from build123d import *

# Parameters (mm, degrees)
SKETCH_R              = 66
PAD_DEPTH             = 7
SKETCH001_R           = 30
PAD001_DEPTH          = 15
PAD002_DEPTH          = 15
POCKET_DEPTH          = 7
POLARPATTERN_COUNT    = 4
FILLET_R              = 10
FILLET001_R           = 2
SKETCH004_R           = 6
POCKET001_DEPTH       = 37.001
SKETCH005_R           = 23
POCKET002_DEPTH       = 10
SKETCH006_R           = 4
POCKET003_DEPTH       = 4
POLARPATTERN001_COUNT = 4
SKETCH007_R           = 2.25
POCKET004_DEPTH       = 535.079942
POLARPATTERN002_COUNT = 4
CHAMFER_SIZE          = 1
SKETCH008_R           = 4
POCKET005_DEPTH       = 37.001


with BuildPart() as part:
    # Sketch → Pad (new body)
    with BuildSketch(Plane.XY):
        Circle(SKETCH_R)
    extrude(amount=PAD_DEPTH)

    # Sketch001 (on Face3 of Pad) → Pad001 (join)
    with BuildSketch(Plane.XY.offset(7)):
        Circle(SKETCH001_R)
    extrude(amount=PAD001_DEPTH)

    # Sketch002 (on Face5 of Pad001) → Pad002 (join)
    with BuildSketch(Plane.XY.offset(22)):
        with BuildLine():
            ThreePointArc((0.3, 14.997), (-15, 0), (0.3, -14.997))
            Line((0.3, -14.997), (150.24, -11.9976))
            ThreePointArc((150.24, -11.9976), (162, 0), (150.24, 11.9976))
            Line((0.3, 14.997), (150.24, 11.9976))
        make_face()
    extrude(amount=PAD002_DEPTH)

    # Sketch003 (on Face3 of Pad002) → Pocket (cut)
    with BuildSketch(Plane.XY.offset(7)):
        with BuildLine():
            ThreePointArc((-6, 49.638695), (-35.355339, 35.355339), (-49.638695, 6))
            Line((-33.76825, 6), (-49.638695, 6))
            ThreePointArc((-6, 33.636641), (-24.113209, 24.067543), (-33.76825, 6))
            Line((-6, 33.636641), (-6, 49.638695))
        make_face()
    pocket = extrude(amount=-POCKET_DEPTH, mode=Mode.SUBTRACT)

    # PolarPattern: Pocket ×4 about axis
    polarpattern_axis = Axis((0, 0, 0), (0, 0, 1))
    for i in range(1, POLARPATTERN_COUNT):
        add(pocket.rotate(polarpattern_axis, i * 360 / POLARPATTERN_COUNT), mode=Mode.SUBTRACT)

    # Fillet
    fillet_edges = [part.edges().sort_by_distance(p)[0] for p in [
        (-30, 0, 22),
    ]]
    fillet(fillet_edges, radius=FILLET_R)

    # Fillet001
    fillet001_edges = [part.edges().sort_by_distance(p)[0] for p in [
        (-33.636641, -6, 3.5),
        (-49.638695, -6, 3.5),
        (-66, 0, 7),
        (-49.638695, 6, 3.5),
        (-6, 49.638695, 3.5),
        (-6, -33.76825, 3.5),
        (-6, -49.638695, 3.5),
        (6, -49.638695, 3.5),
        (6, -33.636641, 3.5),
        (33.76825, -6, 3.5),
        (49.638695, -6, 3.5),
        (49.638695, 6, 3.5),
        (6, 49.638695, 3.5),
        (6, 33.76825, 3.5),
        (33.636641, 6, 3.5),
        (-6, 33.636641, 3.5),
        (-33.76825, 6, 3.5),
        (75.27, -13.4973, 37),
        (-15, 0, 37),
        (75.27, 13.4973, 37),
        (162, 0, 37),
        (88.257783, 13.237492, 22),
        (162, 0, 22),
        (88.257783, -13.237492, 22),
        (-30, 0, 12),
    ]]
    fillet(fillet001_edges, radius=FILLET001_R)

    # Sketch004 (on Face50 of Fillet001) → Pocket001 (cut, through all)
    with BuildSketch(Plane.XY.offset(37)):
        Circle(SKETCH004_R)
    extrude(amount=-POCKET001_DEPTH, mode=Mode.SUBTRACT)

    # Sketch005 (on Face51 of Pocket001) → Pocket002 (cut)
    with BuildSketch(Plane(origin=(0, 0, 0), x_dir=(1, 0, 0), z_dir=(0, 0, -1))):
        with Locations((0.306212, -0.34782)):
            Circle(SKETCH005_R)
    extrude(amount=-POCKET002_DEPTH, mode=Mode.SUBTRACT)

    # Sketch006 (on Face5 of Pocket002) → Pocket003 (cut)
    with BuildSketch(Plane.XY.offset(7)):
        with Locations((-42.376377, 42.476376)):
            Circle(SKETCH006_R)
    pocket003 = extrude(amount=-POCKET003_DEPTH, mode=Mode.SUBTRACT)

    # PolarPattern001: Pocket003 ×4 about axis
    polarpattern001_axis = Axis((0, 0, 0), (0, 0, 1))
    for i in range(1, POLARPATTERN001_COUNT):
        add(pocket003.rotate(polarpattern001_axis, i * 360 / POLARPATTERN001_COUNT), mode=Mode.SUBTRACT)

    # Sketch007 (on Face57 of PolarPattern001) → Pocket004 (cut, through all)
    with BuildSketch(Plane.XY.offset(3)):
        with Locations((-42.376377, 42.476376)):
            Circle(SKETCH007_R)
    pocket004 = extrude(amount=-POCKET004_DEPTH, mode=Mode.SUBTRACT)

    # PolarPattern002: Pocket004 ×4 about axis
    polarpattern002_axis = Axis((0, 0, 0), (0, 0, 1))
    for i in range(1, POLARPATTERN002_COUNT):
        add(pocket004.rotate(polarpattern002_axis, i * 360 / POLARPATTERN002_COUNT), mode=Mode.SUBTRACT)

    # Chamfer
    chamfer_edges = [part.edges().sort_by_distance(p)[0] for p in [
        (-6, 0, 37),
    ]]
    chamfer(chamfer_edges, length=CHAMFER_SIZE)

    # Sketch008 (on Face1 of Chamfer) → Pocket005 (cut, through all)
    with BuildSketch(Plane.XY.offset(37)):
        with Locations((150, 0)):
            Circle(SKETCH008_R)
    extrude(amount=-POCKET005_DEPTH, mode=Mode.SUBTRACT)


solid = part.part
Verification items for the finished model (mm, model axes). A direction names the side the tool comes from. Coordinates: 2 decimals unless noted, no trailing zeros. Write each loop counter-clockwise with the first axis right and the second up, starting at its lowest first coordinate (ties: lowest second). Pieces come first, ordered by that corner, then holes. Notation, with made-up numbers: (64, -11) -> (114, -11) arc R19 ccw to (114, 8) -> close; hole circle Ø2 at (41.5, -19). An arc over 180 degrees is marked (long way). One line per item, written item: value. Start each with the question number.
Q1. Go/stop test with flat-tipped pins: P1, Ø1.5, axis at x = 47.5, y = 22.5, coming from the +Z side; P2, Ø8, axis at y = 6, z = 24.5, coming from the -X side; P3, Ø7, axis at x = 42.48, y = 42.38, coming from the +Z side; P4, Ø8, axis at x = -40.5, z = 14.5, coming from the +Y side. Record where each tip stops, or that it passes through.
Q2. Cross-section at A-A on z = 27.5. Enter the section's corners in (x, y), and give its area (3 significant figures).
Q3. Thickness scan on L1, parallel to X at y = -17, z = 4; L2, parallel to Y at x = 150, z = 31.25; L3, parallel to X at y = 7, z = 5. Record the ranges inside material, lowest first. Write a range as from..to.
Q4. Access from +Z, -Z, +X, -X, +Y, -Y to the whole of each face (thin tool, end or side, straight path). Record for faces 1 (the flat face through (-6, 41, 4)), 2 (the flat face through (-40.65, 40.75, 3)), 3 (the cylindrical face through (74.208, 12.917, 36.43)), 4 (the cylindrical face through (-4.68, 22.8, 4.93)).
Q5. Mould release check, pull along Z, two halves, no side actions. Record for faces 5 (the flat face through (72, 0, 37)), 6 (the flat face through (93, 0, 22)), 7 (the cylindrical face through (-35.66, -35.05, 3.55)): pulls with the +Z half, pulls with the -Z half, needs draft (parallel to the pull), parting line crosses it, or undercut.
Checked values:
1. P1: stops at z = 7
1. P2: stops at x = -24.61
1. P3: stops at z = 3
1. P4: passes through
2. outline: (0.3, -15) -> (150.24, -12) arc R12 ccw to (150.24, 12) -> (0.3, 15) arc R15 ccw (long way) to start; hole circle Ø12 at (0, 0); hole circle Ø8 at (150, 0)
2. area: 4,470 mm²
3. L1: x = -63.77..-47.02, -29.53..-14.8, 15.41..29.59, 47.02..63.77
3. L2: y = -12..-4, 4..12
3. L3: x = -65.63..-49.06, -33.64..-21.71, 22.32..33.52, 49.06..65.63
4. face 1: +Z, -Z
4. face 2: +Z
4. face 3: +Z, +X, +Y
4. face 4: -Z
5. face 5: pulls with the +Z half
5. face 6: undercut
5. face 7: needs draft
